Could you check a few things on this model? Use its own coordinates, in mm. Give positions to 0.01 mm unless a question says otherwise; leave off trailing zeros. Write item = value, one per line. Start each with the question number.
1) I want a section at A-A (y = -287.5). Count the separate pieces of the cut face and the enclosed holes in it, and give its area (3 significant figures).
2) I'm going to push flat-ended pins straight in: pin 1 Ø3 at (y, z) = (-367, -1.5) entering from +X; pin 2 Ø6 at (x, y) = (0, -157.5) entering from -Z; pin 3 Ø5 at (y, z) = (-252.5, 1) entering from +X; pin 4 Ø8 at (x, z) = (-1, -6) entering from +Y. Where does each tip first touch, or does it pass through?
3) I need wall thicknesses on probe 1 along Z at (x, y) = (0, -107); probe 2 along Z at (x, y) = (6.5, -140.5); probe 3 along X at (y, z) = (-130.5, 0.5). Which ranges of each line are inside material? Lowest first, please. Write a range as from..to.
from build123d import *

# Parameters (mm, degrees)
F0_R     = 2.0955
F2_DEPTH = 478


with BuildPart() as f2:
    # F0 (on Front) → F2 (new body)
    with BuildSketch(Plane.XZ):
        with BuildLine():
            Line((-4.6246692655, 9.9949), (-9.0043, 9.9949))
            ThreePointArc((-9.0043, 9.9949), (-9.7047599774, 9.7047599774), (-9.9949, 9.0043))
            Line((-9.9949, 9.0043), (-9.9949, 4.6246692655))
            Line((-9.9949, 4.6246692655), (-8.1915, 2.8212692655))
            Line((-8.1915, 2.8212692655), (-8.1915, 5.4628692655))
            Line((-8.1915, 5.4628692655), (-6.5405, 5.4628692655))
            Line((-6.5405, 5.4628692655), (-3.8989, 2.8212692655))
            Line((-3.8989, 2.8212692655), (-3.8989, -2.8212692655))
            Line((-3.8989, -2.8212692655), (-6.5405, -5.4628692655))
            Line((-6.5405, -5.4628692655), (-8.1915, -5.4628692655))
            Line((-8.1915, -5.4628692655), (-8.1915, -2.8212692655))
            Line((-8.1915, -2.8212692655), (-9.9949, -4.6246692655))
            Line((-9.9949, -4.6246692655), (-9.9949, -9.0043))
            ThreePointArc((-9.9949, -9.0043), (-9.7047599774, -9.7047599774), (-9.0043, -9.9949))
            Line((-9.0043, -9.9949), (-4.6246692655, -9.9949))
            Line((-4.6246692655, -9.9949), (-2.8212692655, -8.1915))
            Line((-2.8212692655, -8.1915), (-5.4628692655, -8.1915))
            Line((-5.4628692655, -8.1915), (-5.4628692655, -6.5405))
            Line((-5.4628692655, -6.5405), (-2.8212692655, -3.8989))
            Line((-2.8212692655, -3.8989), (2.8212692655, -3.8989))
            Line((2.8212692655, -3.8989), (5.4628692655, -6.5405))
            Line((5.4628692655, -6.5405), (5.4628692655, -8.1915))
            Line((5.4628692655, -8.1915), (2.8212692655, -8.1915))
            Line((2.8212692655, -8.1915), (4.6246692655, -9.9949))
            Line((4.6246692655, -9.9949), (9.0043, -9.9949))
            ThreePointArc((9.0043, -9.9949), (9.7047599774, -9.7047599774), (9.9949, -9.0043))
            Line((9.9949, -9.0043), (9.9949, -4.6246692655))
            Line((9.9949, -4.6246692655), (8.1915, -2.8212692655))
            Line((8.1915, -2.8212692655), (8.1915, -5.4628692655))
            Line((8.1915, -5.4628692655), (6.5405, -5.4628692655))
            Line((6.5405, -5.4628692655), (3.8989, -2.8212692655))
            Line((3.8989, -2.8212692655), (3.8989, 2.8212692655))
            Line((3.8989, 2.8212692655), (6.5405, 5.4628692655))
            Line((6.5405, 5.4628692655), (8.1915, 5.4628692655))
            Line((8.1915, 5.4628692655), (8.1915, 2.8212692655))
            Line((8.1915, 2.8212692655), (9.9949, 4.6246692655))
            Line((9.9949, 4.6246692655), (9.9949, 9.0043))
            ThreePointArc((9.9949, 9.0043), (9.7047599774, 9.7047599774), (9.0043, 9.9949))
            Line((9.0043, 9.9949), (4.6246692655, 9.9949))
            Line((4.6246692655, 9.9949), (2.8212692655, 8.1915))
            Line((2.8212692655, 8.1915), (5.4628692655, 8.1915))
            Line((5.4628692655, 8.1915), (5.4628692655, 6.5405))
            Line((5.4628692655, 6.5405), (2.8212692655, 3.8989))
            Line((2.8212692655, 3.8989), (-2.8212692655, 3.8989))
            Line((-2.8212692655, 3.8989), (-5.4628692655, 6.5405))
            Line((-5.4628692655, 6.5405), (-5.4628692655, 8.1915))
            Line((-5.4628692655, 8.1915), (-2.8212692655, 8.1915))
            Line((-2.8212692655, 8.1915), (-4.6246692655, 9.9949))
        make_face()
        with BuildLine():
            ThreePointArc((-8.0391, -8.1915), (-8.1468630735, -8.1468630735), (-8.1915, -8.0391))
            Line((-8.1915, -8.0391), (-8.1915, -6.6929))
            ThreePointArc((-8.1915, -6.6929), (-8.1468630735, -6.5851369265), (-8.0391, -6.5405))
            Line((-8.0391, -6.5405), (-7.9883, -6.5405))
            Line((-7.9883, -6.5405), (-6.5405, -7.9883))
            Line((-6.5405, -7.9883), (-6.5405, -8.0391))
            ThreePointArc((-6.5405, -8.0391), (-6.5851369265, -8.1468630735), (-6.6929, -8.1915))
            Line((-6.6929, -8.1915), (-8.0391, -8.1915))
        make_face(mode=Mode.SUBTRACT)
        with BuildLine():
            Line((8.1915, -6.6929), (8.1915, -8.0391))
            ThreePointArc((8.1915, -8.0391), (8.1468630735, -8.1468630735), (8.0391, -8.1915))
            Line((8.0391, -8.1915), (6.6929, -8.1915))
            ThreePointArc((6.6929, -8.1915), (6.5851369265, -8.1468630735), (6.5405, -8.0391))
            Line((6.5405, -8.0391), (6.5405, -7.9883))
            Line((6.5405, -7.9883), (7.9883, -6.5405))
            Line((7.9883, -6.5405), (8.0391, -6.5405))
            ThreePointArc((8.0391, -6.5405), (8.1468630735, -6.5851369265), (8.1915, -6.6929))
        make_face(mode=Mode.SUBTRACT)
        with BuildLine():
            Line((-7.9883, 6.5405), (-8.0391, 6.5405))
            ThreePointArc((-8.0391, 6.5405), (-8.1468630735, 6.5851369265), (-8.1915, 6.6929))
            Line((-8.1915, 6.6929), (-8.1915, 8.0391))
            ThreePointArc((-8.1915, 8.0391), (-8.1468630735, 8.1468630735), (-8.0391, 8.1915))
            Line((-8.0391, 8.1915), (-6.6929, 8.1915))
            ThreePointArc((-6.6929, 8.1915), (-6.5851369265, 8.1468630735), (-6.5405, 8.0391))
            Line((-6.5405, 8.0391), (-6.5405, 7.9883))
            Line((-6.5405, 7.9883), (-7.9883, 6.5405))
        make_face(mode=Mode.SUBTRACT)
        Circle(F0_R, mode=Mode.SUBTRACT)
        with BuildLine():
            ThreePointArc((8.1915, 6.6929), (8.1468630735, 6.5851369265), (8.0391, 6.5405))
            Line((8.0391, 6.5405), (7.9883, 6.5405))
            Line((7.9883, 6.5405), (6.5405, 7.9883))
            Line((6.5405, 7.9883), (6.5405, 8.0391))
            ThreePointArc((6.5405, 8.0391), (6.5851369265, 8.1468630735), (6.6929, 8.1915))
            Line((6.6929, 8.1915), (8.0391, 8.1915))
            ThreePointArc((8.0391, 8.1915), (8.1468630735, 8.1468630735), (8.1915, 8.0391))
            Line((8.1915, 8.0391), (8.1915, 6.6929))
        make_face(mode=Mode.SUBTRACT)
    extrude(amount=F2_DEPTH)


solid = f2.part
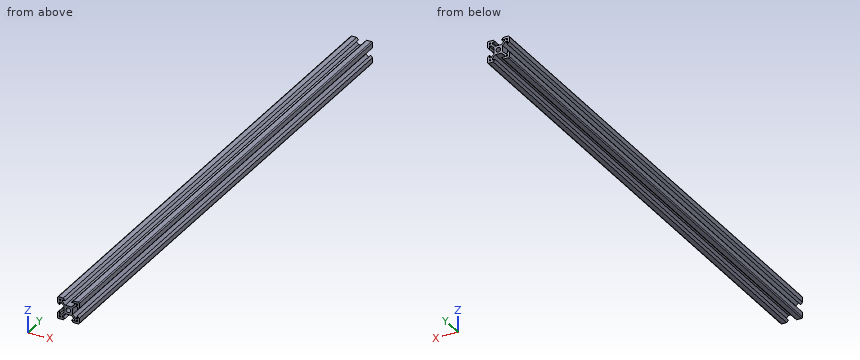
Answer list:
q1.separate_pieces = 1
q1.enclosed_holes = 5
q1.area = 165 mm^2
q2.pin_1 = 8.37
q2.pin_2 = -8.37
q2.pin_3 = 8.87
q2.pin_4 = 0
q3.probe_1 = -3.9..-2.1, 2.1..3.9
q3.probe_2 = -9.99..-5.42, 5.42..9.99
q3.probe_3 = -3.9..-2.03, 2.03..3.9
